Read the model definition and answer for the solid it produces. Units are mm, in the model's axes. Face numbers are marked on the shaded views. A direction names the side the tool comes from. Give positions to 0.01 mm unless a question says otherwise; leave off trailing zeros. Loops run counter-clockwise (first coordinate to the right, second up) from the corner with the lowest first, then second, coordinate; pieces in that order, holes last. Notation, with made-up numbers: (24.5, 12) - (59.5, 12) arc R5 cw to (59.5, 21) - close; hole circle Ø1 at (-7, 16.5). An arc over 180 degrees is marked (long way). Use a Markdown table: item, result. Add a question column.
Item 1: A cutting plane is placed at B-B (y = 33.5). Determine the outline of the cut face in (x, z), plus the area to 3 significant figures.
Item 2: A cutting plane is placed at A-A (x = 30). Determine the outline of the cut face in (y, z), plus the area to 3 significant figures.
Item 3: Each of these flat-tipped pins is pushed along its axis until it touches: P1, Ø2, axis at y = 35, z = 3, coming from the -X side; P2, Ø6, axis at x = 27, y = 9, coming from the +Z side; P3, Ø6, axis at y = 20.5, z = 4, coming from the -X side. Where does it stop, or does it pass through?
Item 4: Consider probe 1 along Y at (x, z) = (27.25, -3); probe 2 along Z at (x, y) = (30, 29.5); probe 3 along Y at (x, z) = (30.5, 2). Determine where each line is inside the solid, lowest interval first. Write a range as [from, to].
Item 5: Which of the six approach directions +Z, -Z, +X, -X, +Y, -Y give full straight-line access (tool end or side, diameter ignored) to the marked faces 1 and 2?
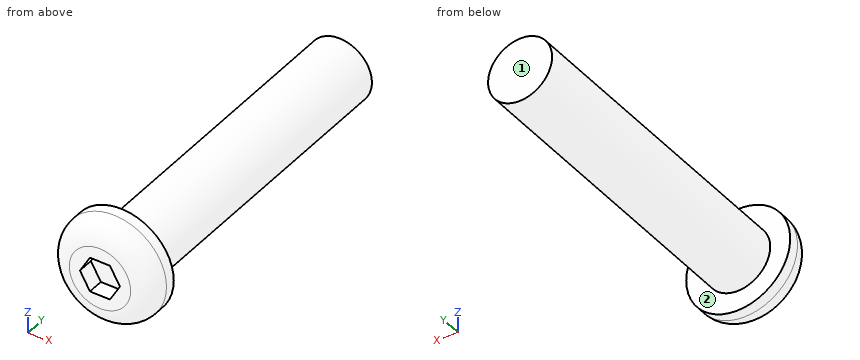
from build123d import *

# Parameters (mm, degrees)
SKETCH_1_W          = 6.5
SKETCH_1_H          = 4
SKETCH_2_R          = 4
EXTRUDE_1_DEPTH     = 40
CUT_EXTRUDE_1_DEPTH = 2
FILLET_1_R          = 2.666666667


with BuildPart() as part:
    # 草图1 → 旋转1 (revolve)
    with BuildSketch(Plane.XY):
        with Locations((33.25, 2)):
            Rectangle(SKETCH_1_W, SKETCH_1_H)
    revolve(axis=Axis((30, 4, 0), (0, -1, 0)))

    # 草图2 → 凸台-拉伸1 (add)
    with BuildSketch(Plane(origin=(0, 4, 0), x_dir=(-1, 0, 0), z_dir=(0, 1, 0))):
        with Locations((-30, 0)):
            Circle(SKETCH_2_R)
    extrude(amount=EXTRUDE_1_DEPTH)

    # 草图3 → 切除-拉伸1 (cut)
    with BuildSketch(Plane.XZ):
        Polygon((28.75, -2.165063509), (31.25, -2.165063509), (32.5, 0), (31.25, 2.165063509), (28.75, 2.165063509), (27.5, 0), align=None)
    extrude(amount=-CUT_EXTRUDE_1_DEPTH, mode=Mode.SUBTRACT)

    # 圆角1
    fillet_1_edges = [part.edges().sort_by_distance(p)[0] for p in [
        (23.5, 0, 0),
    ]]
    fillet(fillet_1_edges, radius=FILLET_1_R)


solid = part.part
Geometry says:
| question | item | result |
|---|---|---|
| 1 | outline | circle Ø8 at (30, 0) |
| 1 | area | 50.3 mm² |
| 2 | outline | (0, -3.83) arc R2.67 ccw to (2.67, -6.5) - (4, -6.5) - (4, -4) - (44, -4) - (44, 4) - (4, 4) - (4, 6.5) - (2.67, 6.5) arc R2.67 ccw to (0, 3.83) - (0, 2.17) - (2, 2.17) - (2, -2.17) - (0, -2.17) - close |
| 2 | area | 360 mm² |
| 3 | P1 | x = 26.54 |
| 3 | P2 | z = 4 |
| 3 | P3 | x = 26.13 |
| 4 | probe 1 | [0.01, 4] |
| 4 | probe 2 | [-4, 4] |
| 4 | probe 3 | [2, 44] |
| 5 | face 1 | +Z, -Z, +X, -X, +Y |
| 5 | face 2 | +Y |
